```python
from build123d import *

# Parameters (mm, degrees)
F1_DEPTH = 60
F0_W     = 84.12575
F0_H     = 57.152696
F2_DEPTH = 60
F3_T     = -2.5
F4_W     = 22
F4_H     = 54
F5_DEPTH = 5


with BuildPart() as f1:
    # F0 (on Right) → F1 (new body, symmetric)
    with BuildSketch(Plane.YZ):
        Polygon((-42.062875, -28.576348), (-42.062875, 28.576348), (-84.691621, -28.576348), align=None)
    extrude(amount=F1_DEPTH, both=True)

    # F0 (on Right) → F2 (join, symmetric)
    with BuildSketch(Plane.YZ):
        Rectangle(F0_W, F0_H)
        Polygon((-42.062875, -28.576348), (-42.062875, 28.576348), (-84.691621, -28.576348), align=None)
    extrude(amount=F2_DEPTH, both=True)

    # F3
    f3_openings = [f1.faces().sort_by_distance(p)[0] for p in [
        (0, 0, 28.576348),
    ]]
    offset(amount=F3_T, openings=f3_openings)

    # F4 (on face) → F5 (cut)
    with BuildSketch(Plane(origin=(0, 0, -28.576348), x_dir=(1, 0, 0), z_dir=(0, 0, -1))):
        with Locations((-40, 50)):
            Rectangle(F4_W, F4_H)
        with Locations((40, 50)):
            Rectangle(F4_W, F4_H)
    extrude(amount=-F5_DEPTH, mode=Mode.SUBTRACT)


solid = f1.part
```
Here's how the part is built. I have some questions about the finished solid (model axes, mm). A direction names the side the tool comes from. Give positions to 0.01 mm unless a question says otherwise; leave off trailing zeros. Order: outer loops, then holes, each group sorted by start corner. A loop starts at its lowest first (then second) coordinate and runs counter-clockwise, first axis right, second up. Notation, with made-up numbers: M -27,9.5 L 6,9.5 A22 ccw 6,39.5 Z; hole C 43,-3.5 d1. An arc over 180 degrees is marked long. Use a Markdown table: item, result. Add a question column.
1. Suppose I cut it at D-D (y = 23.5). List the corners of the cut face in (x, z) for me, and give its area (3 significant figures).
2. If we mould it in two halves opening along Y, with no side actions, what happens to faces 1 (the flat face through (1, 39.563, 1)), 2 (the flat face through (0.84, -63.08, 0.4)), 3 (the flat face through (57.5, -8, 2)), 4 (the flat face through (-60, -8, 0))? For each: +Y half, -Y half, draft (parallel to the pull), parting line (faces both ways), or undercut.
3. For pin 1 Ø1.5 at (x, y) = (-43.5, -62) entering from -Z; pin 2 Ø1 at (x, z) = (44, -4) entering from -Y; pin 3 Ø16.5 at (x, z) = (-17, -7) entering from -Y, each with a flat end and sliding along its axis, tell me the tip position at first contact or that it passes through.
4. Suppose I cut it at B-B (x = 46). List the corners of the cut face in (y, z) for me.
5. Suppose I cut it at A-A (y = -34). List the corners of the cut face in (x, z) for me.
6. On a 3-axis mill with a long thin cutter (end or side, diameter ignored), from which of +Z, -Z, +X, -X, +Y, -Y can I reach the whole of each face in a straight line? I mean faces 5 (the flat face through (1, -22, -28.576)), 6 (the flat face through (0.805, -59.041, 1.633)). Say none if no direction works.
7. I need wall thicknesses on probe 1 along X at (y, z) = (30.5, -13); probe 2 along Z at (x, y) = (-3, -23); probe 3 along Y at (x, z) = (-9, 7.5). Which ranges of each line are inside material? Lowest first, please. Write a range as from..to.
8. Suppose I cut it at C-C (z = 19.5). List the corners of the cut face in (x, y) for me.
Results list:
| question | item | result |
|---|---|---|
| 1 | outline | M -60,-28.58 L 60,-28.58 L 60,28.58 L 57.5,28.58 L 57.5,-26.08 L -57.5,-26.08 L -57.5,28.58 L -60,28.58 Z |
| 1 | area | 573 mm² |
| 2 | face 1 | undercut |
| 2 | face 2 | -Y half |
| 2 | face 3 | undercut |
| 2 | face 4 | draft |
| 3 | pin 1 | stops at z = -3.34 |
| 3 | pin 2 | stops at y = -66.73 |
| 3 | pin 3 | stops at y = -74.75 |
| 4 | outline | M -84.69,-28.58 L -77,-28.58 L -77,-26.08 L -79.71,-26.08 L -38.94,28.58 L -42.06,28.58 Z; M -23,-28.58 L 42.06,-28.58 L 42.06,28.58 L 39.56,28.58 L 39.56,-26.08 L -23,-26.08 Z |
| 5 | outline | M -60,-28.58 L -51,-28.58 L -51,-26.08 L -57.5,-26.08 L -57.5,28.58 L -60,28.58 Z; M -29,-28.58 L 29,-28.58 L 29,-26.08 L -29,-26.08 Z; M 51,-28.58 L 60,-28.58 L 60,28.58 L 57.5,28.58 L 57.5,-26.08 L 51,-26.08 Z |
| 6 | face 5 | -Z, +X, -X, +Y, -Y |
| 6 | face 6 | none |
| 7 | probe 1 | x = -60..-57.5, 57.5..60 |
| 7 | probe 2 | z = -28.58..-26.08 |
| 7 | probe 3 | y = -57.78..-54.66, 39.56..42.06 |
| 8 | outline | M -60,-48.83 L 60,-48.83 L 60,42.06 L -60,42.06 Z; hole M -57.5,-45.71 L 57.5,-45.71 L 57.5,39.56 L -57.5,39.56 Z |
